Answer from the drawing. Dimensions are ordinates in mm from the lowest x, y and z of the part. A direction names the side the tool comes from. Coordinates: 2 decimals unless noted, no trailing zeros. Order: outer loops, then holes, each group sorted by start corner. A loop starts at its lowest first (then second) coordinate and runs counter-clockwise, first axis right, second up. Notation, with made-up numbers: M -9.5,-3.75 L 9.5,-3.75 A25 ccw 9.5,13.25 Z; hole C -38,31.25 d9. An arc over 180 degrees is marked long. Write each question's results on one line, items separated by ' | '.
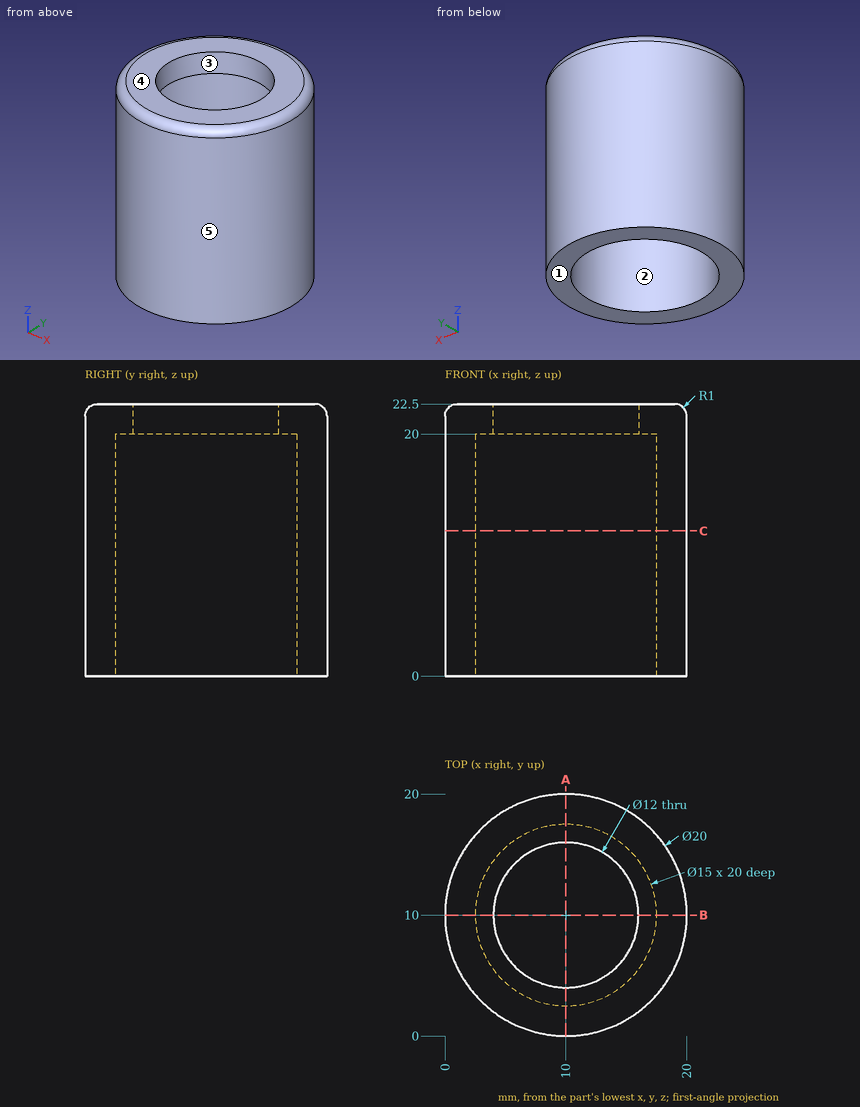
(1) For the marked faces 1 and 2, determine the directions among +Z, -Z, +X, -X, +Y, -Y from which every point of the face is accessible in a straight line to the end or side of a thin tool.
Conclusion:
face 1: -Z, +X, -X, +Y, -Y | face 2: -Z
(2) Straight lines are drawn through the part: line 1 (Y direction, x = 10, z = 6.5); line 2 (Y direction, x = 10, z = 21.2); line 3 (X direction, y = 8.5, z = 17.5). For each, find the intervals that lie inside material, in ascending order.
Conclusion:
line 1: 0 to 2.5, 17.5 to 20 | line 2: 0 to 4, 16 to 20 | line 3: 0.11 to 2.65, 17.35 to 19.89
(3) The mould has two halves that part along X. Classify the marked faces 3, 4 and 5: pulls with the +X half, pulls with the -X half, needs draft (parallel to the pull), parting line crosses it, or undercut.
Conclusion:
face 3: undercut | face 4: needs draft | face 5: parting line crosses it
(4) Given pin 1 (2 mm diameter, centred on x = 16.5, z = 19.5, fed in from -Y); pin 2 (1.5 mm diameter, centred on x = 18, z = 10.5, fed in from -Y); pin 3 (4 mm diameter, centred on x = 15.5, z = 20, fed in from -Y), each flat-ended and moving along its own axis, determine where each tip first touches the part or whether it passes through.
Conclusion:
pin 1: y = 1.65 | pin 2: y = 3.11 | pin 3: y = 0.63
(5) The part is cut by section C-C, the plane z = 12. Write down the section's boundary in (x, y), then the cut area to 3 significant figures.
Conclusion:
outline: C 10,10 d20; hole C 10,10 d15 | area: 137 mm²
(6) The part is cut by section A-A, the plane x = 10. Write down the section's boundary in (y, z).
Conclusion:
outline: M 0,0 L 2.5,0 L 2.5,20 L 4,20 L 4,22.5 L 1,22.5 A1 ccw 0,21.5 Z; M 16,20 L 17.5,20 L 17.5,0 L 20,0 L 20,21.5 A1 ccw 19,22.5 L 16,22.5 Z
